Geometry check sheet. Reference: the model listing, model coordinates, mm. Face numbers are marked on the shaded views. A direction names the side the tool comes from. Give positions to 0.01 mm unless a question says otherwise; leave off trailing zeros. Write each loop counter-clockwise with the first axis right and the second up, starting at its lowest first coordinate (ties: lowest second). Pieces come first, ordered by that corner, then holes. Notation, with made-up numbers: M 74.5,61.25 L 92.5,61.25 A31 ccw 92.5,93.25 Z; hole C 74.25,-16 d8. An arc over 180 degrees is marked long. Write each question's results on one line, items separated by ' | '.
```python
from build123d import *

# Parameters (mm, degrees)
BOSS_EXTRUDE1_DEPTH = 9.144
BOSS_EXTRUDE7_START = 2.54
SKETCH3_W           = 5.497965662
SKETCH3_H           = 5.686621346
SKETCH3_W_2         = 2.537497481
SKETCH3_H_2         = 2.494515015
BOSS_EXTRUDE7_DEPTH = 2.54
BOSS_EXTRUDE8_DEPTH = 9.144
SKETCH9_W           = 9.68799942
SKETCH9_H           = 2.539743385
BOSS_EXTRUDE9_DEPTH = 3.175


with BuildPart() as part:
    # Sketch2 → Boss-Extrude1 (new body)
    with BuildSketch(Plane(origin=(0, 0, 0), x_dir=(1, 0, 0), z_dir=(0, 1, 0))):
        with BuildLine():
            Line((-16.484821535, 14.991226562), (19.965175413, 14.992229827))
            ThreePointArc((19.965175413, 14.992229827), (34.453763808, 16.669641544), (32.919177794, 2.165230163))
            ThreePointArc((32.919177794, 2.165230163), (34.454264788, -12.338688941), (19.966174864, -10.660770051))
            Line((19.966174864, -10.660770051), (6.526477702, -10.661139971))
            Line((6.526477702, -10.661139971), (6.526477702, -13.201139972))
            Line((6.526477702, -13.201139972), (18.666916826, -13.200805813))
            ThreePointArc((18.666916826, -13.200805813), (35.566435216, -14.762300874), (36.785563248, 2.165360379))
            ThreePointArc((36.785563248, 2.165360379), (35.565859505, 19.093319416), (18.665967138, 17.532194068))
            Line((18.665967138, 17.532194068), (-15.185563688, 17.531262324))
            ThreePointArc((-15.185563688, 17.531262324), (-32.085077033, 19.092756448), (-33.30420747, 2.165100491))
            ThreePointArc((-33.30420747, 2.165100491), (-32.08450617, -14.762857534), (-15.184614497, -13.201737557))
            Line((-15.184614497, -13.201737557), (-3.161521718, -13.201406628))
            Line((-3.161521718, -13.201406628), (-3.161521718, -10.661406627))
            Line((-3.161521718, -10.661406627), (-16.483822084, -10.661773316))
            ThreePointArc((-16.483822084, -10.661773316), (-30.972409917, -12.339179924), (-29.437822557, 2.165230163))
            ThreePointArc((-29.437822557, 2.165230163), (-29.581379954, 2.259029678), (-29.723191237, 2.355448738))
            ThreePointArc((-29.723191237, 2.355448738), (-30.849950106, 16.788680298), (-16.484821535, 14.991226562))
        make_face()
    extrude(amount=-BOSS_EXTRUDE1_DEPTH)

    # Sketch3 → Boss-Extrude7 (add)
    with BuildSketch(Plane(origin=(0, 0, 0), x_dir=(-1, 0, 0), z_dir=(0, 1, 0)).offset(BOSS_EXTRUDE7_START)):
        with BuildLine():
            Line((-6.526477702, 13.201139972), (-18.666916826, 13.200805813))
            ThreePointArc((-18.666916826, 13.200805813), (-35.566435216, 14.762300874), (-36.785563248, -2.165360379))
            ThreePointArc((-36.785563248, -2.165360379), (-35.565859505, -19.093319416), (-18.665967138, -17.532194068))
            Line((-18.665967138, -17.532194068), (15.185563688, -17.531262324))
            ThreePointArc((15.185563688, -17.531262324), (32.085077033, -19.092756448), (33.30420747, -2.165100491))
            ThreePointArc((33.30420747, -2.165100491), (32.08450617, 14.762857534), (15.184614497, 13.201737557))
            Line((15.184614497, 13.201737557), (3.161521718, 13.201406628))
            Line((3.161521718, 13.201406628), (-6.526477702, 13.201406628))
            Line((-6.526477702, 13.201406628), (-6.526477702, 13.201139972))
        make_face()
        Polygon((16.725192045, 3.202079604), (20.733260983, 3.202079604), (20.733260983, -3.35074569), (32.292495251, -3.35074569), (32.292495251, -7.184972831), (20.037093812, -7.184972831), (20.037093812, -5.761606936), (16.725192045, -5.761606936), align=None, mode=Mode.SUBTRACT)
        with Locations((-28.472988633, 8.375990138)):
            Rectangle(SKETCH3_W, SKETCH3_H, mode=Mode.SUBTRACT)
        with Locations((29.691821719, 2.533771638)):
            Rectangle(SKETCH3_W_2, SKETCH3_H_2, mode=Mode.SUBTRACT)
    extrude(amount=-BOSS_EXTRUDE7_DEPTH)

    # Sketch8 → Boss-Extrude8 (add)
    with BuildSketch(Plane.XZ):
        with BuildLine():
            Line((-16.484821535, -14.991226562), (19.965175413, -14.992229827))
            Line((19.965175413, -14.992229827), (19.965175413, -12.452229827))
            Line((19.965175413, -12.452229827), (-33.422355561, -12.452229827))
            ThreePointArc((-33.422355561, -12.452229827), (-25.785203294, -19.26939309), (-16.484821535, -14.991226562))
        make_face()
        with BuildLine():
            Line((19.965175413, -12.452229827), (19.965175413, -14.992229827))
            ThreePointArc((19.965175413, -14.992229827), (29.266220586, -19.269979209), (36.903423899, -12.452229827))
            Line((36.903423899, -12.452229827), (26.676938614, -12.452229827))
            Line((26.676938614, -12.452229827), (19.965175413, -12.452229827))
        make_face()
        with BuildLine():
            Line((26.676938614, -12.452229827), (36.903423899, -12.452229827))
            ThreePointArc((36.903423899, -12.452229827), (36.591930347, -6.6578073), (32.919177794, -2.165230163))
            Line((32.919177794, -2.165230163), (26.676938614, -2.165230163))
            Line((26.676938614, -2.165230163), (26.676938614, -12.452229827))
        make_face()
        Polygon((19.966174864, 8.137271719), (19.966174864, 10.660770051), (7.41756795, 10.661115444), (7.41756795, 8.137271719), align=None)
    extrude(amount=BOSS_EXTRUDE8_DEPTH)

    # Sketch9 → Boss-Extrude9 (add)
    with BuildSketch(Plane.XZ):
        with Locations((1.682477992, 11.93127832)):
            Rectangle(SKETCH9_W, SKETCH9_H)
    extrude(amount=BOSS_EXTRUDE9_DEPTH)


solid = part.part
```
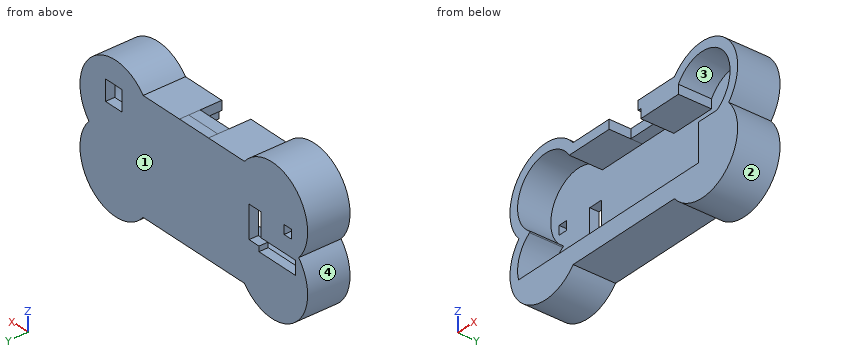
Q1. Depth check by flat-ended pin: P1, Ø1.3, axis at y = 1.5, z = 7, coming from the +X side; P2, Ø1, axis at y = -4.5, z = -0.5, coming from the -X side; P3, Ø2, axis at x = -30, y = 1.5, coming from the +Z side. Enter the tip coordinate at first touch or a pass-through.
Answer key:
P1: stops at x = 39.75 | P2: stops at x = -34.82 | P3: stops at z = 16.66
Q2. Section check C-C (y = 1.5). State how many separate pieces and enclosed holes the cut face has, then the cut area to 3 significant figures.
Answer key:
separate pieces: 1 | enclosed holes: 3 | area: 2,390 mm2
Q3. Access from +Z, -Z, +X, -X, +Y, -Y to the whole of each face (thin tool, end or side, straight path). Record for the marked faces 3 and 4.
Answer key:
face 3: -Y | face 4: +Y, -Y
Q4. Section check D-D (x = 34.5). Enter the section's corners in (y, z), then the cut area to 3 significant figures.
Answer key:
outline: M -9.14,-19.9 L 2.54,-19.9 L 2.54,15.57 L -9.14,15.57 L -9.14,12.29 L 0,12.29 L 0,-0.89 L -9.14,-0.89 Z | area: 294 mm2
Q5. Section check A-A (z = -0.5). Enter the section's corners in (x, y).
Answer key:
outline: M -34.53,-9.14 L -31.39,-9.14 L -31.39,0 L -20.73,0 L -20.73,2.54 L -34.53,2.54 Z; M -16.73,0 L 34.87,0 L 34.87,-9.14 L 38.02,-9.14 L 38.02,2.54 L -16.73,2.54 Z
Q6. Section check B-B (x = -25). Enter the section's corners in (y, z), then the cut area to 3 significant figures.
Answer key:
outline: M -9.14,-21.9 L 2.54,-21.9 L 2.54,-7.18 L 0,-7.18 L 0,-12.45 L -9.14,-12.45 Z; M -9.14,15.02 L 0,15.02 L 0,-3.35 L 2.54,-3.35 L 2.54,17.57 L -9.14,17.57 Z | area: 200 mm2
Q7. Release check for a two-part mould opening along Z. For the marked faces 1 and 2 record: released by +Z, released by -Z, zero draft, split by the parting line, or undercut.
Answer key:
face 1: zero draft | face 2: undercut
Q8. Material ranges on probe 1 along X at (y, z) = (-6.75, -10.5); probe 2 along Z at (x, y) = (6.5, -1); probe 3 along Z at (x, y) = (-27, -3.75), recorded low to high. Write a range as [from, to].
Answer key:
probe 1: x = [-36.27, -33.73], [26.68, 39.75] | probe 2: z = [-17.53, -12.45], [10.66, 13.2] | probe 3: z = [-21.62, -12.45], [14.67, 17.29]
